Design review of the part built by this model. Coordinates are the model's own, in mm. A direction names the side the tool comes from. Round coordinates to 2 decimals unless told otherwise and drop trailing zeros. Write each loop counter-clockwise with the first axis right and the second up, starting at its lowest first coordinate (ties: lowest second). Pieces come first, ordered by that corner, then holes. Notation, with made-up numbers: (79.5, 83) -> (130.5, 83) arc R21 ccw to (130.5, 117) -> close; hole circle Ø9 at (-1, 10). An arc over 180 degrees is marked (long way). Write item = value, one per line. Start each with the question number.
Item 1: Add section A-A, the plane x = 0. State the section outline as (y, z) points.
Item 2: Add section B-B, the plane z = -3. State the section outline as (x, y) points, then the cut area to 3 significant figures.
Item 3: To check wall thickness, follow L1, parallel to Z at x = 3, y = 48.05 (3 decimals); L2, parallel to Y at x = -7.75, z = 4; L3, parallel to X at y = 22, z = 6. State the ranges of each line that lie inside material, in increasing order.
Item 4: For pin 1 Ø6 at (x, z) = (-1, -0.5) entering from -Y; pin 2 Ø3 at (y, z) = (28, 8) entering from -X, all flat-tipped, find the tip position at first contact; note any pin that passes through.
Item 5: Add section C-C, the plane y = 8. State the section outline as (x, z) points, then the cut area to 3 significant figures.
Item 6: Mouldability with a two-part tool opening along Y and no side actions: class faces 3 (the flat face through (-12.25, 1, 0)), 4 (the flat face through (0, 49, 0)), 5 (the flat face through (0, 0, 0)), 6 (the flat face through (-4, 47, 0)) as released by +Y, released by -Y, zero draft, split by the parting line, or undercut.
Item 7: Machinability: for faces 1 (the flat face through (11, 24, -11.25)), 2 (the flat face through (-4, 2, 0)), which of the approach directions +Z, -Z, +X, -X, +Y, -Y give a long, thin tool a straight path to every point of the face, cutting with its end or side? Answer none if there is none.
from build123d import *

# Parameters (mm, degrees)
SKETCH1_W            = 24.5
SKETCH1_H            = 22.5
BOSS_EXTRUDE1_DEPTH  = 2
SKETCH2_W            = 2
SKETCH2_H            = 22.5
BOSS_EXTRUDE2_DEPTH  = 45
SKETCH4_W            = 24.5
SKETCH4_H            = 22.5
BOSS_EXTRUDE3_DEPTH  = 2
SKETCH3_R            = 0.375
CUT_EXTRUDE1_DEPTH   = 50
LPATTERN1_COUNT      = 5
LPATTERN1_PITCH      = 4
LPATTERN1_COUNT_DIR2 = 5
LPATTERN1_PITCH_DIR2 = 4


with BuildPart() as part:
    # Sketch1 → Boss-Extrude1 (new body)
    with BuildSketch(Plane(origin=(0, 0, 0), x_dir=(1, 0, 0), z_dir=(0, 1, 0))):
        Rectangle(SKETCH1_W, SKETCH1_H)
    extrude(amount=BOSS_EXTRUDE1_DEPTH)

    # Sketch2 → Boss-Extrude2 (add)
    with BuildSketch(Plane(origin=(0, 2, 0), x_dir=(1, 0, 0), z_dir=(0, 1, 0))):
        with Locations((11.25, 0)):
            Rectangle(SKETCH2_W, SKETCH2_H)
    extrude(amount=BOSS_EXTRUDE2_DEPTH)

    # Sketch4 → Boss-Extrude3 (add)
    with BuildSketch(Plane(origin=(0, 47, 0), x_dir=(1, 0, 0), z_dir=(0, 1, 0))):
        Rectangle(SKETCH4_W, SKETCH4_H)
    extrude(amount=BOSS_EXTRUDE3_DEPTH)

    # Sketch3 → Cut-Extrude1 (cut, through all)
    with BuildSketch(Plane.XZ):
        with Locations((-9, 8)):
            Circle(SKETCH3_R)
    cut_extrude1 = extrude(amount=-CUT_EXTRUDE1_DEPTH, mode=Mode.SUBTRACT)

    # LPattern1: Cut-Extrude1 5 × 5
    with Locations(*[(j * LPATTERN1_PITCH_DIR2, 0, -i * LPATTERN1_PITCH) for i in range(LPATTERN1_COUNT) for j in range(LPATTERN1_COUNT_DIR2) if (i, j) != (0, 0)]):
        add(cut_extrude1, mode=Mode.SUBTRACT)


solid = part.part
Result set:
q1.outline = (0, -11.25) -> (2, -11.25) -> (2, 11.25) -> (0, 11.25) -> close; (47, -11.25) -> (49, -11.25) -> (49, 11.25) -> (47, 11.25) -> close
q2.outline = (-12.25, 0) -> (12.25, 0) -> (12.25, 49) -> (-12.25, 49) -> (-12.25, 47) -> (10.25, 47) -> (10.25, 2) -> (-12.25, 2) -> close
q2.area = 188 mm²
q3.L1 = -11.25 to -8.375, -7.625 to -4.375, -3.625 to -0.375, 0.375 to 3.625, 4.375 to 7.625, 8.375 to 11.25
q3.L2 = 0 to 2, 47 to 49
q3.L3 = 10.25 to 12.25
q4.pin_1 = 0
q4.pin_2 = 10.25
q5.outline = (10.25, -11.25) -> (12.25, -11.25) -> (12.25, 11.25) -> (10.25, 11.25) -> close
q5.area = 45.0 mm²
q6.face_3 = zero draft
q6.face_4 = released by +Y
q6.face_5 = released by -Y
q6.face_6 = undercut
q7.face_1 = -Z, +X, -X, +Y, -Y
q7.face_2 = +Z, -Z, -X
